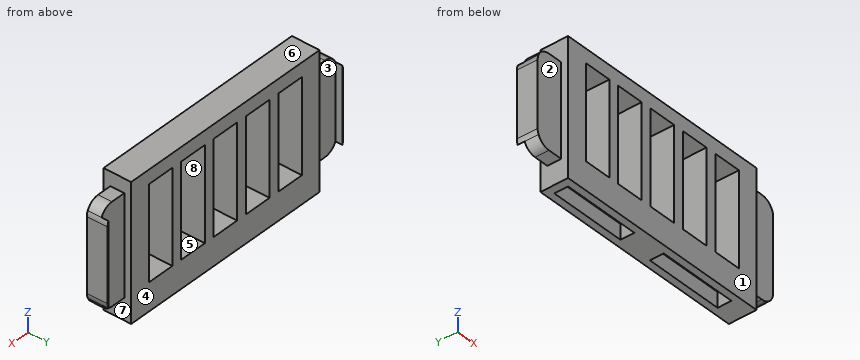
from build123d import *

# Parameters (mm, degrees)
F0_W     = 8
F0_H     = 26.900017
F0_H_2   = 26.905365
F1_DEPTH = 6
F2_DEPTH = 2
F3_DEPTH = 8
F4_W     = 23
F4_H     = 4
F4_W_2   = 22.5
F5_DEPTH = 5


with BuildPart() as f1:
    # F0 (on Front) → F1 (new body)
    with BuildSketch(Plane.XZ):
        with BuildLine():
            Line((-85.422808, 9.222019), (-85.422808, 31.025267))
            ThreePointArc((-85.422808, 31.025267), (-85.64706, 30.296735), (-85.722808, 29.538243))
            Line((-85.722808, 29.538243), (-85.722808, 10.709043))
            ThreePointArc((-85.722808, 10.709043), (-85.64706, 9.950551), (-85.422808, 9.222019))
        make_face()
        with BuildLine():
            ThreePointArc((-5.722808, 31.73826), (-5.798556, 32.496752), (-6.022808, 33.225284))
            Line((-6.022808, 33.225284), (-6.022808, 9.222019))
            ThreePointArc((-6.022808, 9.222019), (-5.798556, 9.950551), (-5.722808, 10.709043))
            Line((-5.722808, 10.709043), (-5.722808, 31.73826))
        make_face()
        with BuildLine():
            Line((-9.558208, 35.57366), (-13.722808, 35.57366))
            Line((-13.722808, 35.57366), (-13.722808, 8.673643))
            Line((-13.722808, 8.673643), (-13.722808, 6.873643))
            Line((-13.722808, 6.873643), (-9.558208, 6.873643))
            ThreePointArc((-9.558208, 6.873643), (-7.436068, 7.514232), (-6.022808, 9.222019))
            Line((-6.022808, 9.222019), (-6.022808, 33.225284))
            ThreePointArc((-6.022808, 33.225284), (-7.436068, 34.93307), (-9.558208, 35.57366))
        make_face()
        Polygon((-71.722808, 39.57366), (-77.722808, 39.57366), (-77.722808, 35.57366), (-77.722808, 33.373643), (-77.722808, 15.555412), (-77.722808, 8.673643), (-77.722808, 6.873643), (-77.722808, 0.673643), (-71.722808, 0.673643), (-13.722808, 0.673643), (-13.722808, 6.873643), (-13.722808, 8.673643), (-13.722808, 35.57366), (-13.722808, 39.57366), (-21.722808, 39.57366), align=None)
        with Locations((-67.722808, 22.123651)):
            Rectangle(F0_W, F0_H, mode=Mode.SUBTRACT)
        with Locations((-56.722808, 22.123651)):
            Rectangle(F0_W, F0_H, mode=Mode.SUBTRACT)
        with Locations((-45.722808, 22.123651)):
            Rectangle(F0_W, F0_H, mode=Mode.SUBTRACT)
        with Locations((-34.722808, 22.123651)):
            Rectangle(F0_W, F0_H, mode=Mode.SUBTRACT)
        with Locations((-23.722808, 22.124238)):
            Rectangle(F0_W, F0_H_2, mode=Mode.SUBTRACT)
        with BuildLine():
            Line((-77.722808, 15.555412), (-77.722808, 33.373643))
            Line((-77.722808, 33.373643), (-81.887408, 33.373643))
            ThreePointArc((-81.887408, 33.373643), (-84.009549, 32.733053), (-85.422808, 31.025267))
            Line((-85.422808, 31.025267), (-85.422808, 9.222019))
            ThreePointArc((-85.422808, 9.222019), (-84.009549, 7.514232), (-81.887408, 6.873643))
            Line((-81.887408, 6.873643), (-77.722808, 6.873643))
            Line((-77.722808, 6.873643), (-77.722808, 8.673643))
            Line((-77.722808, 8.673643), (-77.722808, 15.555412))
        make_face()
    extrude(amount=F1_DEPTH)

    # F0 (on Front) → F2 (cut)
    with BuildSketch(Plane.XZ):
        with BuildLine():
            Line((-77.722808, 15.555412), (-77.722808, 33.373643))
            Line((-77.722808, 33.373643), (-81.887408, 33.373643))
            ThreePointArc((-81.887408, 33.373643), (-84.009549, 32.733053), (-85.422808, 31.025267))
            Line((-85.422808, 31.025267), (-85.422808, 9.222019))
            ThreePointArc((-85.422808, 9.222019), (-84.009549, 7.514232), (-81.887408, 6.873643))
            Line((-81.887408, 6.873643), (-77.722808, 6.873643))
            Line((-77.722808, 6.873643), (-77.722808, 8.673643))
            Line((-77.722808, 8.673643), (-77.722808, 15.555412))
        make_face()
        with BuildLine():
            Line((-9.558208, 35.57366), (-13.722808, 35.57366))
            Line((-13.722808, 35.57366), (-13.722808, 8.673643))
            Line((-13.722808, 8.673643), (-13.722808, 6.873643))
            Line((-13.722808, 6.873643), (-9.558208, 6.873643))
            ThreePointArc((-9.558208, 6.873643), (-7.436068, 7.514232), (-6.022808, 9.222019))
            Line((-6.022808, 9.222019), (-6.022808, 33.225284))
            ThreePointArc((-6.022808, 33.225284), (-7.436068, 34.93307), (-9.558208, 35.57366))
        make_face()
    extrude(amount=F2_DEPTH, mode=Mode.SUBTRACT)

    # F0 (on Front) → F3 (join)
    with BuildSketch(Plane.XZ):
        Polygon((-71.722808, 39.57366), (-77.722808, 39.57366), (-77.722808, 35.57366), (-77.722808, 33.373643), (-77.722808, 15.555412), (-77.722808, 8.673643), (-77.722808, 6.873643), (-77.722808, 0.673643), (-71.722808, 0.673643), (-13.722808, 0.673643), (-13.722808, 6.873643), (-13.722808, 8.673643), (-13.722808, 35.57366), (-13.722808, 39.57366), (-21.722808, 39.57366), align=None)
        with Locations((-67.722808, 22.123651)):
            Rectangle(F0_W, F0_H, mode=Mode.SUBTRACT)
        with Locations((-56.722808, 22.123651)):
            Rectangle(F0_W, F0_H, mode=Mode.SUBTRACT)
        with Locations((-45.722808, 22.123651)):
            Rectangle(F0_W, F0_H, mode=Mode.SUBTRACT)
        with Locations((-34.722808, 22.123651)):
            Rectangle(F0_W, F0_H, mode=Mode.SUBTRACT)
        with Locations((-23.722808, 22.124238)):
            Rectangle(F0_W, F0_H_2, mode=Mode.SUBTRACT)
    extrude(amount=F3_DEPTH)

    # F4 (on Top) → F5 (cut)
    with BuildSketch(Plane.XY):
        Polygon((-75.366058, -1.990048), (-75.366058, -5.990048), (-52.866058, -5.990048), (-52.866058, -3.990048), (-52.866058, -1.990048), align=None)
        Polygon((-42.866058, -1.990048), (-42.866058, -5.990048), (-19.866058, -5.990048), (-19.866058, -3.990048), (-19.866058, -1.990048), align=None)
        with Locations((23.633942, -3.990048)):
            Rectangle(F4_W, F4_H)
        with Locations((56.383942, -3.990048)):
            Rectangle(F4_W_2, F4_H)
    extrude(amount=F5_DEPTH, mode=Mode.SUBTRACT)


solid = f1.part
Model file for the job. Use its own axes, mm. Face numbers are marked on the shaded views. A direction names the side the tool comes from. Give positions to 0.01 mm unless a question says otherwise; leave off trailing zeros. Write each loop counter-clockwise with the first axis right and the second up, starting at its lowest first coordinate (ties: lowest second). Pieces come first, ordered by that corner, then holes. Notation, with made-up numbers: (76, 10.5) - (131, 10.5) arc R32 ccw to (131, 39.5) - close; hole circle Ø10 at (62, 83). An arc over 180 degrees is marked (long way). Answer as CSV lines item,"result".
1. Pin check, flat tips, straight feed: pin 1 (1.2 mm diameter, centred on x = -10.5, y = -3.5, fed in from -Z); pin 2 (2 mm diameter, centred on x = -38, y = -3.5, fed in from -Z). Stop position of each tip, or through.
Responses:
pin 1,"stops at z = 6.87"
pin 2,"stops at z = 5"
2. Two-plate mould, pull along Z, no slides. Class the marked faces 6, 7 and 8: +Z half, -Z half, draft (parallel to the pull), parting line (faces both ways), or undercut.
Responses:
face 6,"+Z half"
face 7,"draft"
face 8,"undercut"
3. Band-saw the part on A-A (x = -47). Write the cut outline in (y, z).
Responses:
outline,"(-8, 0.67) - (0, 0.67) - (0, 8.67) - (-8, 8.67) - close; (-8, 35.57) - (0, 35.57) - (0, 39.57) - (-8, 39.57) - close"
4. Band-saw the part on C-C (z = 3). Write the cut outline in (x, y), and give its area (3 significant figures).
Responses:
outline,"(-77.72, -8) - (-13.72, -8) - (-13.72, 0) - (-77.72, 0) - close; hole (-75.37, -5.99) - (-52.87, -5.99) - (-52.87, -1.99) - (-75.37, -1.99) - close; hole (-42.87, -5.99) - (-19.87, -5.99) - (-19.87, -1.99) - (-42.87, -1.99) - close"
area,"330 mm2"
5. 3-axis set-ups, long thin cutter, end or side, ignore diameter. For the marked faces 1, 2, 3, 4 and 5: which of +Z, -Z, +X, -X, +Y, -Y reach the whole face in a straight line?
Responses:
face 1,"+Z, -Z, +X, -X, -Y"
face 2,"+Z, -Z, -X, -Y"
face 3,"+Z, -Z, +Y"
face 4,"+Z, -Z, +X, -X, +Y"
face 5,"+Y, -Y"
6. Drill centre lines: L1, parallel to X at y = -3, z = 22.5; L2, parallel to X at y = -4.75, z = 4; L3, parallel to X at y = -7.5, z = 22.5. Where is each one in solid material? Low to high. Write a range as [from, to].
Responses:
L1,"x = [-85.72, -71.72], [-63.72, -60.72], [-52.72, -49.72], [-41.72, -38.72], [-30.72, -27.72], [-19.72, -5.72]"
L2,"x = [-77.72, -75.37], [-52.87, -42.87], [-19.87, -13.72]"
L3,"x = [-77.72, -71.72], [-63.72, -60.72], [-52.72, -49.72], [-41.72, -38.72], [-30.72, -27.72], [-19.72, -13.72]"
7. Band-saw the part on B-B (y = -1). Count the separate pieces of the cut face and the enclosed holes in it, and give its area (3 significant figures).
Responses:
separate pieces,"3"
enclosed holes,"5"
area,"1,430 mm2"
8. Band-saw the part on D-D (y = -7). Write the cut outline in (x, z), and give its area (3 significant figures).
Responses:
outline,"(-77.72, 0.67) - (-13.72, 0.67) - (-13.72, 39.57) - (-77.72, 39.57) - close; hole (-71.72, 8.67) - (-63.72, 8.67) - (-63.72, 35.57) - (-71.72, 35.57) - close; hole (-60.72, 8.67) - (-52.72, 8.67) - (-52.72, 35.57) - (-60.72, 35.57) - close; hole (-49.72, 8.67) - (-41.72, 8.67) - (-41.72, 35.57) - (-49.72, 35.57) - close; hole (-38.72, 8.67) - (-30.72, 8.67) - (-30.72, 35.57) - (-38.72, 35.57) - close; hole (-27.72, 8.67) - (-19.72, 8.67) - (-19.72, 35.58) - (-27.72, 35.58) - close"
area,"1,410 mm2"
